Can you work these out from the model? Positions are in its coordinate system, mm. Face numbers are marked on the shaded views. A direction names the side the tool comes from. Give positions to 0.01 mm unless a question says otherwise; leave off trailing zeros. Order: outer loops, then holes, each group sorted by start corner. A loop starts at its lowest first (then second) coordinate and runs counter-clockwise, first axis right, second up. Notation, with made-up numbers: (-13, 73) - (-5, 73) arc R19 ccw to (-5, 77) - close; hole circle Ø9 at (61, 47). An arc over 180 degrees is marked (long way). Use one line per item in the form item = value. Start each with the question number.
1) Suppose I cut it at D-D, the plane y = -2.5. Write out the boundary of the cut face in (x, z) (3 decimals).
2) Please list where these lines run through material, in increasing order: probe 1 along Y at (x, z) = (38.1, 2); probe 2 along X at (y, z) = (-1.25, 6); probe 3 along Z at (x, y) = (39, 1.75) (3 decimals).
3) Suppose I cut it at A-A, the plane z = 2.5. State how many separate pieces and enclosed holes the cut face has, and give its area (3 significant figures).
4) Suppose I cut it at C-C, the plane y = 1. Write out the boundary of the cut face in (x, z) (3 decimals).
5) Which directions (+Z, -Z, +X, -X, +Y, -Y) give clear straight access to the entire face, cutting with the end or side of a thin tool? Please do the marked faces 4 and 5.
6) We'd pull the mould along X, two halves only. Please class the marked faces 1, 2 and 3: released by +X, released by -X, zero draft, split by the parting line, or undercut.
7) For pin 1 (3 mm diameter, centred on x = 0, y = 0, fed in from -Z), with a flat end and sliding along its axis, tell me the tip position at first contact or that it passes through.
8) Suppose I cut it at B-B, the plane x = -1. Write out the boundary of the cut face in (y, z).
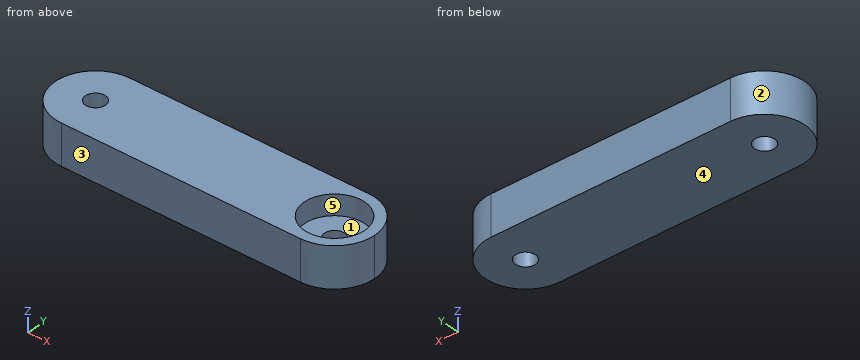
```python
from build123d import *

# Parameters (mm, degrees)
F0_R     = 1.5875
F1_DEPTH = 6.35
F2_R     = 4.7625
F3_DEPTH = 3.175


with BuildPart() as f1:
    # F0 (on Top) → F1 (new body)
    with BuildSketch(Plane.XY):
        with BuildLine():
            ThreePointArc((0, 6.35), (4.490128, 4.490128), (6.35, 0))
            ThreePointArc((6.35, 0), (4.490128, -4.490128), (0, -6.35))
            Line((0, -6.35), (38.1, -6.35))
            ThreePointArc((38.1, -6.35), (31.75, 0), (38.1, 6.35))
            Line((38.1, 6.35), (0, 6.35))
        make_face()
        with BuildLine():
            ThreePointArc((44.45, 0), (42.590128, 4.490128), (38.1, 6.35))
            ThreePointArc((38.1, 6.35), (31.75, 0), (38.1, -6.35))
            ThreePointArc((38.1, -6.35), (42.590128, -4.490128), (44.45, 0))
        make_face()
        with Locations((38.1, 0)):
            Circle(F0_R, mode=Mode.SUBTRACT)
        with BuildLine():
            ThreePointArc((0, -6.35), (4.490128, -4.490128), (6.35, 0))
            ThreePointArc((6.35, 0), (4.490128, 4.490128), (0, 6.35))
            ThreePointArc((0, 6.35), (-6.35, 0), (0, -6.35))
        make_face()
        Circle(F0_R, mode=Mode.SUBTRACT)
    extrude(amount=F1_DEPTH)

    # F2 (on face) → F3 (cut)
    with BuildSketch(Plane.XY.offset(6.35)):
        with Locations((38.1, 0)):
            Circle(F2_R)
    extrude(amount=-F3_DEPTH, mode=Mode.SUBTRACT)


solid = f1.part
```
Result sheet:
q1.outline = (-5.837, 0) - (43.937, 0) - (43.937, 6.35) - (42.154, 6.35) - (42.154, 3.175) - (34.046, 3.175) - (34.046, 6.35) - (-5.837, 6.35) - close
q2.probe_1 = -6.35 to -1.59, 1.59 to 6.35
q2.probe_2 = -6.23 to -0.98, 0.98 to 33.5, 42.7 to 44.33
q2.probe_3 = 0 to 3.175
q3.separate_pieces = 1
q3.enclosed_holes = 2
q3.area = 595 mm²
q4.outline = (-6.271, 0) - (-1.233, 0) - (-1.233, 6.35) - (-6.271, 6.35) - close; (1.233, 0) - (36.867, 0) - (36.867, 3.175) - (33.444, 3.175) - (33.444, 6.35) - (1.233, 6.35) - close; (39.333, 0) - (44.371, 0) - (44.371, 6.35) - (42.756, 6.35) - (42.756, 3.175) - (39.333, 3.175) - close
q5.face_4 = -Z, +X, -X, +Y, -Y
q5.face_5 = +Z
q6.face_1 = undercut
q6.face_2 = released by -X
q6.face_3 = zero draft
q7.pin_1 = through
q8.outline = (-6.27, 0) - (-1.23, 0) - (-1.23, 6.35) - (-6.27, 6.35) - close; (1.23, 0) - (6.27, 0) - (6.27, 6.35) - (1.23, 6.35) - close
